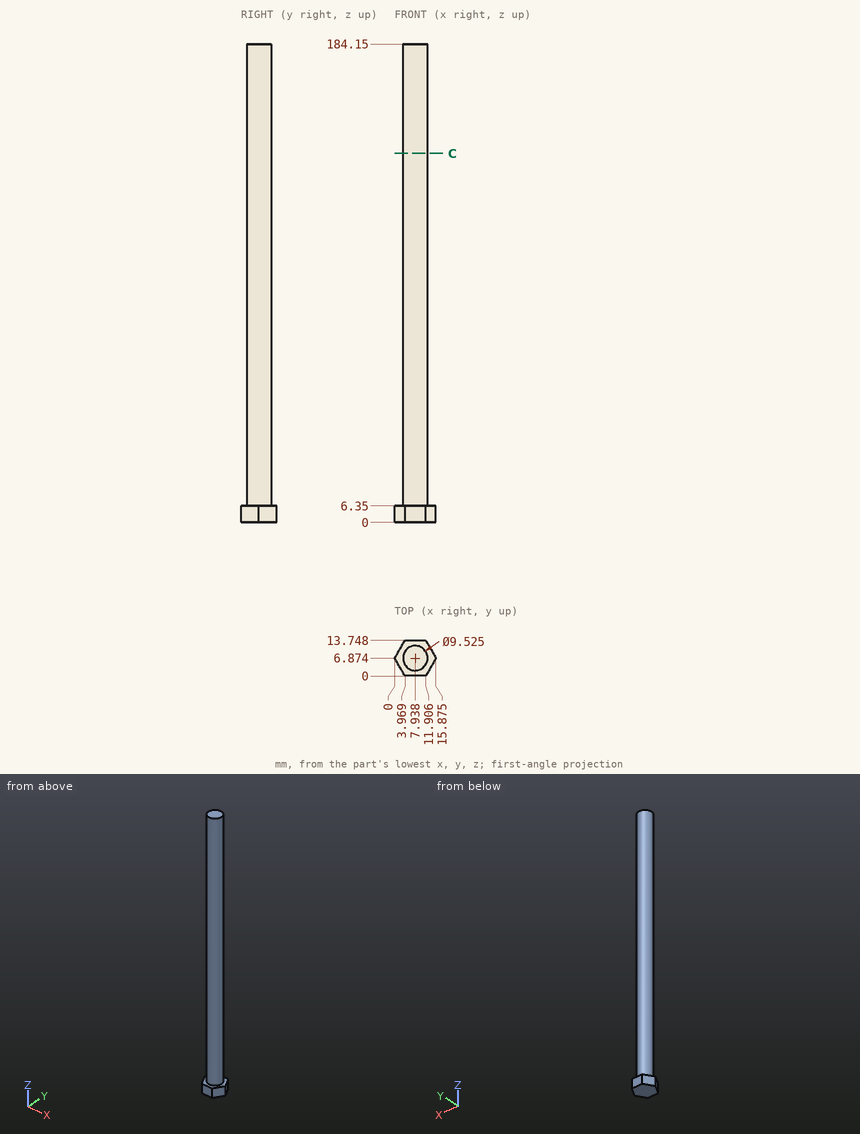
Geometry check sheet. Reference: drawing and pictorial views, mm from the part's lowest x, y, z. Coordinates: 2 decimals unless noted, no trailing zeros. Order: outer loops, then holes, each group sorted by start corner. A loop starts at its lowest first (then second) coordinate and runs counter-clockwise, first axis right, second up.
Item 1: Depth check by flat-ended pin: pin 1 (1 mm diameter, centred on y = 7, z = 37.5, fed in from +X); pin 2 (3 mm diameter, centred on x = 9.5, z = 94.5, fed in from +Y); pin 3 (5 mm diameter, centred on x = 6, z = 28, fed in from -Y). Enter the tip coordinate at first touch or a pass-through.
Item 2: Section check C-C (z = 142). Enter the section's corners in (x, y) (1 decimal).
Item 3: Scan lines: line 1 along Z through (x, y) = (4.75, 12.5); line 2 along Y through (x, z) = (8, 91); line 3 along X through (y, z) = (6.5, 18) (1 decimal). Record each from-to range of solid material in increasing order.
Check sheet entries:
1. pin 1: stops at x = 12.7
1. pin 2: stops at y = 11.64
1. pin 3: stops at y = 2.11
2. outline: circle Ø9.5 at (7.9, 6.9)
3. line 1: z = 0 to 6.35
3. line 2: y = 2.11 to 11.64
3. line 3: x = 3.2 to 12.7
